```python
from build123d import *

# Parameters (mm, degrees)
F0_W = 6.35
F0_H = 12.7


with BuildPart() as f1:
    # F0 (on Top) → F1 (revolve)
    with BuildSketch(Plane.XY):
        Polygon((-5.963771, -11.02523), (-5.963771, 46.12477), (-12.313771, 46.12477), (-21.838771, 46.12477), (-21.838771, -11.02523), align=None)
        Polygon((-5.963771, -30.07523), (-5.963771, -11.02523), (-21.838771, -11.02523), (-40.888771, -11.02523), (-40.888771, -30.07523), align=None)
        with Locations((-9.138771, 52.47477)):
            Rectangle(F0_W, F0_H)
    revolve(axis=Axis((3.561229, 14.37477, 0), (0, -1, 0)))


solid = f1.part
```
For this review, take the finished solid that the model builds, in its own axes (mm). A direction names the side the tool comes from. Coordinates: 2 decimals unless noted, no trailing zeros. Loops run counter-clockwise (first coordinate to the right, second up) from the corner with the lowest first, then second, coordinate; pieces in that order, holes last. Notation, with made-up numbers: (55.5, 78) -> (104.5, 78) arc R21 ccw to (104.5, 83) -> close; hole circle Ø2 at (78.5, -20). An arc over 180 degrees is marked (long way). Return JSON: item names as keys, results as strings. Group by question number.
(1) Consider section C-C, the plane y = -22.5. Give the boundary of the cut face in (x, z) (3 decimals), plus the area to 3 significant figures.
(2) Consider section D-D, the plane x = -11. Give the boundary of the cut face in (y, z), plus the area to 3 significant figures.
(3) Consider section B-B, the plane x = 3.5. Give the boundary of the cut face in (y, z), plus the area to 3 significant figures.
(4) Tool access review of faces 4 (the cylindrical face through (6.868, 17.15, -25.184)), 5 (the flat face through (4, -30.075, -11)): name each direction out of +Z, -Z, +X, -X, +Y, -Y from which nothing blocks a thin tool from reaching the whole face with its end or side.
(5) Consider section A-A, the plane z = 0. Give the boundary of the cut face in (x, y), plus the area to 3 significant figures.
(6) Mouldability with a two-part tool opening along Z and no side actions: class faces 1 (the cylindrical face through (7, 52.6, 15.5)), 2 (the cylindrical face through (-5.237, 14.997, 3.648)), 3 (the flat face through (4, 58.825, 10)) as pulls with the +Z half, pulls with the -Z half, needs draft (parallel to the pull), parting line crosses it, or undercut.
(7) To check wall thickness, follow L1, parallel to X at y = 32.5, z = 0; L2, parallel to Z at x = 11, y = -20; L3, parallel to Z at x = 3, y = 40. State the ranges of each line that lie inside material, in increasing order.
(8) For pin 1 Ø10 at (x, y) = (26.5, 25.5) entering from +Z; pin 2 Ø12 at (y, z) = (19, 9) entering from -X; pin 3 Ø2 at (x, y) = (25.5, -12) entering from -Z, all flat-tipped, find the tip position at first contact; note any pin that passes through.
Results below:
{
 "1": {"outline": "circle Ø88.9 at (3.561, 0); hole circle Ø19.05 at (3.561, 0)", "area": "5,920 mm2"},
 "2": {"outline": "(-30.08, -42) -> (-11.03, -42) -> (-11.03, -20.81) -> (46.12, -20.81) -> (46.12, -6.32) -> (58.82, -6.32) -> (58.82, 6.32) -> (46.12, 6.32) -> (46.12, 20.81) -> (-11.03, 20.81) -> (-11.03, 42) -> (-30.08, 42) -> close", "area": "4,140 mm2"},
 "3": {"outline": "(-30.08, -44.45) -> (-11.03, -44.45) -> (-11.03, -25.4) -> (46.12, -25.4) -> (46.12, -15.87) -> (58.82, -15.87) -> (58.82, -9.52) -> (-30.08, -9.52) -> close; (-30.08, 9.52) -> (58.82, 9.52) -> (58.82, 15.87) -> (46.12, 15.87) -> (46.12, 25.4) -> (-11.03, 25.4) -> (-11.03, 44.45) -> (-30.08, 44.45) -> close", "area": "3,310 mm2"},
 "4": {"face 4": "+Y", "face 5": "+Z, -Z, +X, -X, -Y"},
 "5": {"outline": "(-40.89, -30.08) -> (-5.96, -30.08) -> (-5.96, 58.82) -> (-12.31, 58.82) -> (-12.31, 46.12) -> (-21.84, 46.12) -> (-21.84, -11.03) -> (-40.89, -11.03) -> close; (13.09, -30.08) -> (48.01, -30.08) -> (48.01, -11.03) -> (28.96, -11.03) -> (28.96, 46.12) -> (19.44, 46.12) -> (19.44, 58.82) -> (13.09, 58.82) -> close", "area": "3,310 mm2"},
 "6": {"face 1": "parting line crosses it", "face 2": "undercut", "face 3": "needs draft"},
 "7": {"L1": "x = -21.84 to -5.96, 13.09 to 28.96", "L2": "z = -43.82 to -5.95, 5.95 to 43.82", "L3": "z = -25.39 to -9.51, 9.51 to 25.39"},
 "8": {"pin 1": "stops at z = 17.98", "pin 2": "stops at x = -21.66", "pin 3": "stops at z = -39.21"}
}
